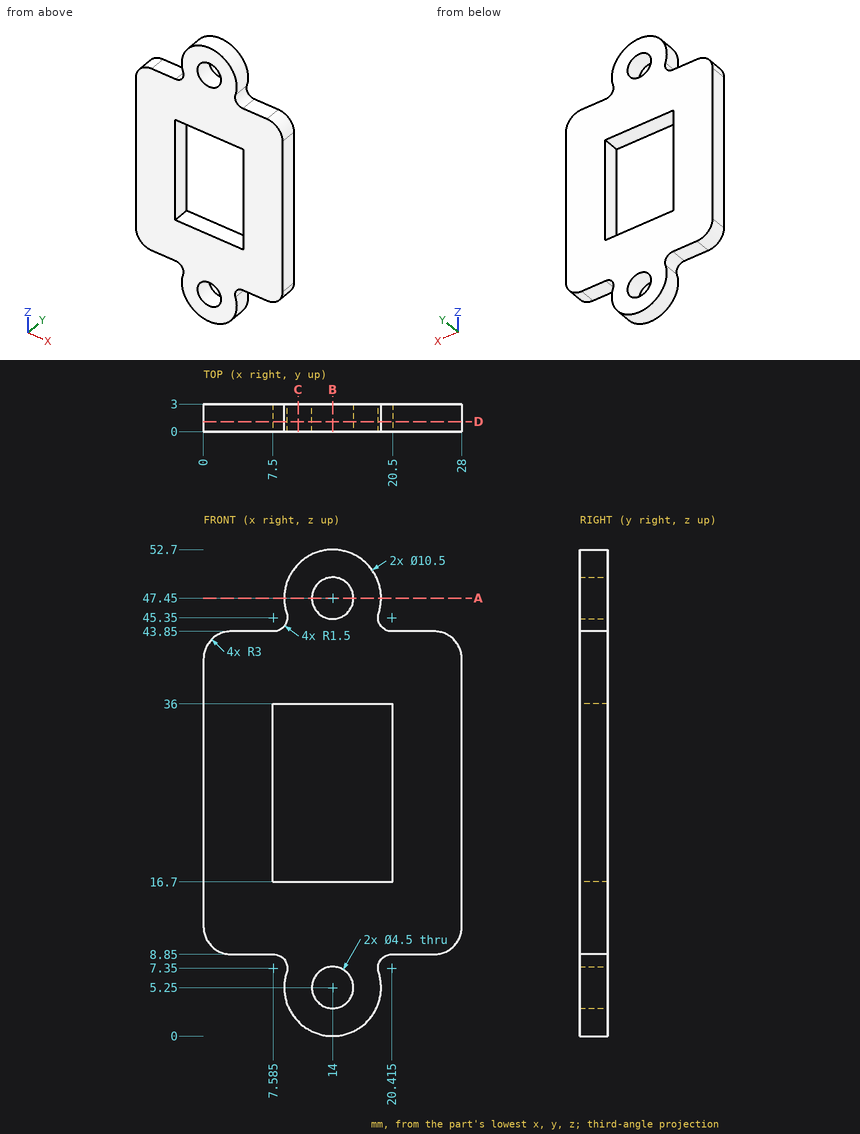
Could you check a few things on this drawing? It's one solid part, dimensions in mm from its lowest x, y, z. Round coordinates to 2 decimals unless told otherwise and drop trailing zeros. Write each loop counter-clockwise with the first axis right and the second up, starting at its lowest first coordinate (ties: lowest second). Pieces come first, ordered by that corner, then holes. Notation, with made-up numbers: (43, 2.5) -> (97, 2.5) arc R32 cw to (97, 31.5) -> close; hole circle Ø8 at (21, -7). An arc over 180 degrees is marked (long way). One line per item, written item: value.
1) Suppose I cut it at B-B on x = 14. List the corners of the cut face in (y, z) for me, plus the area to 3 significant figures.
Filled sheet:
outline: (0, 0) -> (3, 0) -> (3, 3) -> (0, 3) -> close; (0, 7.5) -> (3, 7.5) -> (3, 16.7) -> (0, 16.7) -> close; (0, 36) -> (3, 36) -> (3, 45.2) -> (0, 45.2) -> close; (0, 49.7) -> (3, 49.7) -> (3, 52.7) -> (0, 52.7) -> close
area: 73.2 mm2
2) Suppose I cut it at A-A on z = 47.45. List the corners of the cut face in (x, y) for me, plus the area to 3 significant figures.
Filled sheet:
outline: (8.75, 0) -> (11.75, 0) -> (11.75, 3) -> (8.75, 3) -> close; (16.25, 0) -> (19.25, 0) -> (19.25, 3) -> (16.25, 3) -> close
area: 18.0 mm2
3) If I drill on line 1 (X direction, y = 1.7, z = 35); line 2 (Z direction, x = 15.25, y = 0.2); line 3 (Z direction, x = 6.5, y = 0.9), over which ranges is the centre line in solid material (lowest first)? Write a range as [from, to].
Filled sheet:
line 1: x = [0, 7.5], [20.5, 28]
line 2: z = [0.15, 3.38], [7.12, 16.7], [36, 45.58], [49.32, 52.55]
line 3: z = [8.85, 43.85]
4) Suppose I cut it at D-D on y = 1.1. Give the number of separate pieces and of enclosed holes in the cut face, plus the area to 3 significant figures.
Filled sheet:
separate pieces: 1
enclosed holes: 3
area: 851 mm2
5) I'm going to push flat-ended pins straight in: pin 1 Ø4 at (x, z) = (14, 47.45) entering from +Y; pin 2 Ø0.9 at (x, y) = (4.5, 1) entering from +Z; pin 3 Ø0.9 at (x, y) = (23.5, 2) entering from -Z. Where does each tip first touch, or does it pass through?
Filled sheet:
pin 1: passes through
pin 2: stops at z = 43.85
pin 3: stops at z = 8.85
6) Suppose I cut it at C-C on x = 10.25. List the corners of the cut face in (y, z) for me.
Filled sheet:
outline: (0, 1.58) -> (3, 1.58) -> (3, 16.7) -> (0, 16.7) -> close; (0, 36) -> (3, 36) -> (3, 51.12) -> (0, 51.12) -> close
